Design review of the part built by this model. Coordinates are the model's own, in mm. A direction names the side the tool comes from. Give positions to 0.01 mm unless a question says otherwise; leave off trailing zeros. Loops run counter-clockwise (first coordinate to the right, second up) from the corner with the lowest first, then second, coordinate; pieces in that order, holes last. Notation, with made-up numbers: (89.25, -32) - (102.25, -32) arc R21 cw to (102.25, -6) - close; hole circle Ø10 at (7, 48). An arc over 180 degrees is marked (long way). Write each question's results on one line, items separated by ' | '.
from build123d import *

# Parameters (mm, degrees)
SKETCH1_R             = 30
BOSS_EXTRUDE1_DEPTH   = 10
F_6_0MM_DOWEL_HOLE1_D = 6
SKETCH2_R             = 11
BOSS_EXTRUDE2_DEPTH   = 10
SKETCH9_R             = 3.95
BOSS_EXTRUDE3_DEPTH   = 30


with BuildPart() as part:
    # Sketch1 → Boss-Extrude1 (new body)
    with BuildSketch(Plane.XY):
        Circle(SKETCH1_R)
    extrude(amount=BOSS_EXTRUDE1_DEPTH)

    # Ø6.0mm Dowel Hole1 (through all)
    with Locations(Plane.XY.offset(10)):
        with Locations((-15.733125881, 15.733125881), (15.733125881, -15.733125881), (-15.733125881, -15.733125881)):
            Hole(F_6_0MM_DOWEL_HOLE1_D / 2)

    # Sketch2 → Boss-Extrude2 (add)
    with BuildSketch(Plane.XY.offset(10)):
        Circle(SKETCH2_R)
    extrude(amount=BOSS_EXTRUDE2_DEPTH)

    # Sketch9 → Boss-Extrude3 (add)
    with BuildSketch(Plane.XY.offset(20)):
        with Locations((0, -3)):
            Circle(SKETCH9_R)
    extrude(amount=BOSS_EXTRUDE3_DEPTH)


solid = part.part
(1) Tool access review of faces 4 (the flat face through (0, 0, 0)), 5 (the flat face through (13, 0, 10)): name each direction out of +Z, -Z, +X, -X, +Y, -Y from which nothing blocks a thin tool from reaching the whole face with its end or side.
Answers below:
face 4: -Z, +X, -X, +Y, -Y | face 5: +Z
(2) Take a section at C-C on z = 36. Give the boundary of the cut face in (x, y), plus the area to 3 significant figures.
Answers below:
outline: circle Ø7.9 at (0, -3) | area: 49.0 mm2
(3) Take a section at D-D on x = 6. Give the boundary of the cut face in (y, z).
Answers below:
outline: (-29.39, 0) - (29.39, 0) - (29.39, 10) - (9.22, 10) - (9.22, 20) - (-9.22, 20) - (-9.22, 10) - (-29.39, 10) - close
(4) Insertion check: P1, Ø8, axis at x = 15.73, y = -15.73, coming from the +Z side; P2, Ø6, axis at y = -14.5, z = 11.5, coming from the -X side; P3, Ø8, axis at x = 5, z = 35, coming from the -Y side; P4, Ø10, axis at x = -18.5, z = 24.5, coming from the +Y side. Each pin has a flat end and moves straight along its axis. Give the tip position at first contact, or say it passes through.
Answers below:
P1: z = 10 | P2: x = -27.54 | P3: y = -6.82 | P4: through
(5) Draft analysis for pull direction X (two halves, no side actions). For faces 1 (the cylindrical face through (-2.38, -10.74, 14.93)), 2 (the flat face through (0, 3, 20)), 3 (the cylindrical face through (-13.352, -17.559, 4.93)), state which applies: pulls with the +X half, pulls with the -X half, needs draft (parallel to the pull), parting line crosses it, or undercut.
Answers below:
face 1: parting line crosses it | face 2: needs draft | face 3: undercut
(6) Take a section at A-A on x = 0. Give the boundary of the cut face in (y, z), plus the area to 3 significant figures.
Answers below:
outline: (-30, 0) - (30, 0) - (30, 10) - (11, 10) - (11, 20) - (0.95, 20) - (0.95, 50) - (-6.95, 50) - (-6.95, 20) - (-11, 20) - (-11, 10) - (-30, 10) - close | area: 1,060 mm2
(7) Take a section at B-B on y = -5.5. Give the boundary of the cut face in (x, z).
Answers below:
outline: (-29.49, 0) - (29.49, 0) - (29.49, 10) - (9.53, 10) - (9.53, 20) - (3.06, 20) - (3.06, 50) - (-3.06, 50) - (-3.06, 20) - (-9.53, 20) - (-9.53, 10) - (-29.49, 10) - close
(8) Wall thickness on line 1 along Z through (x, y) = (7.5, 5.5); line 2 along Z through (x, y) = (-25.5, -15); line 3 along Y through (x, z) = (3, 30): over which ranges is each line inside the solid? List them lowest first. Write a range as from..to.
Answers below:
line 1: 0..20 | line 2: 0..10 | line 3: -5.57..-0.43
